from build123d import *

# Parameters (mm, degrees)
F1_DEPTH = 3
F2_W     = 50
F2_H     = 56.5
F3_DEPTH = 25


with BuildPart() as f1:
    # F0 (on Front) → F1 (new body)
    with BuildSketch(Plane.XZ):
        with BuildLine():
            Line((14.135233, 37.539159), (-41.864767, 37.539159))
            ThreePointArc((-41.864767, 37.539159), (-43.986087, 36.660479), (-44.864767, 34.539159))
            Line((-44.864767, 34.539159), (-44.864767, -27.960841))
            ThreePointArc((-44.864767, -27.960841), (-43.986087, -30.082161), (-41.864767, -30.960841))
            Line((-41.864767, -30.960841), (14.135233, -30.960841))
            ThreePointArc((14.135233, -30.960841), (16.256553, -30.082161), (17.135233, -27.960841))
            Line((17.135233, -27.960841), (17.135233, 34.539159))
            ThreePointArc((17.135233, 34.539159), (16.256553, 36.660479), (14.135233, 37.539159))
        make_face()
    extrude(amount=F1_DEPTH)

    # F2 (on face) → F3 (cut)
    with BuildSketch(Plane.XZ.offset(3)):
        with Locations((-13.864767, 3.289159)):
            Rectangle(F2_W, F2_H)
    extrude(amount=-F3_DEPTH, mode=Mode.SUBTRACT)


solid = f1.part
For this review, take the finished solid that the model builds, in its own axes (mm). A direction names the side the tool comes from. Round coordinates to 2 decimals unless told otherwise and drop trailing zeros. Write each loop counter-clockwise with the first axis right and the second up, starting at its lowest first coordinate (ties: lowest second). Pieces come first, ordered by that corner, then holes. Notation, with made-up numbers: (-4, -3.5) - (26, -3.5) arc R30 cw to (26, 32.5) - close; hole circle Ø1 at (82.25, 50.5). An arc over 180 degrees is marked (long way). Write item = value, one per line. Start each with the question number.
1. Consider section B-B on y = -2.5. State the section outline as (x, z) points, plus the area to 3 significant figures.
2. For faces 4 (the face through (-14, -1, -30.961)), 5 (the face through (-38.865, -2, 3)), list the 3-axis set-ups (+Z, -Z, +X, -X, +Y, -Y) from which the entire face can be reached by the end or side of a thin tool; tool diameter is ignored.
3. Consider section C-C on x = -15. State the section outline as (y, z) points.
4. Consider section A-A on z = 5. State the section outline as (x, y) points, plus the area to 3 significant figures.
5. Wall thickness on L1, parallel to Z at x = -17, y = -1.4; L2, parallel to X at y = -0.95, z = -23: over which ranges is each line inside the solid? List them lowest first.
6. Draft analysis for pull direction X (two halves, no side actions). For faces 1 (the face through (-42, -3, 4)), 2 (the face through (-14, -2, 31.539)), 3 (the face through (-44.01, -1.48, -30.06)), state which applies: released by +X, released by -X, zero draft, split by the parting line, or undercut.
7. For pin 1 Ø12 at (x, z) = (-32.5, 29) entering from -Y, flat-tipped, find the tip position at first contact; note if it passes through.
Evaluation:
q1.outline = (-44.86, -27.96) arc R3 ccw to (-41.86, -30.96) - (14.14, -30.96) arc R3 ccw to (17.14, -27.96) - (17.14, 34.54) arc R3 ccw to (14.14, 37.54) - (-41.86, 37.54) arc R3 ccw to (-44.86, 34.54) - close; hole (-38.86, -24.96) - (11.14, -24.96) - (11.14, 31.54) - (-38.86, 31.54) - close
q1.area = 1,410 mm2
q2.face_4 = -Z, +X, -X, +Y, -Y
q2.face_5 = +Y, -Y
q3.outline = (-3, -30.96) - (0, -30.96) - (0, -24.96) - (-3, -24.96) - close; (-3, 31.54) - (0, 31.54) - (0, 37.54) - (-3, 37.54) - close
q4.outline = (-44.86, -3) - (-38.86, -3) - (-38.86, 0) - (-44.86, 0) - close; (11.14, -3) - (17.14, -3) - (17.14, 0) - (11.14, 0) - close
q4.area = 36.0 mm2
q5.L1 = -30.96 to -24.96, 31.54 to 37.54
q5.L2 = -44.86 to -38.86, 11.14 to 17.14
q6.face_1 = zero draft
q6.face_2 = undercut
q6.face_3 = released by -X
q7.pin_1 = -3
